```python
from build123d import *

# Parameters (mm, degrees)
F1_DEPTH = 2
F2_R     = 1
F3_R     = 4
F4_W     = 13.5
F4_H     = 1.8558323957
F5_DEPTH = 5
F6_R     = 1
F7_D     = 1


with BuildPart() as f1:
    # F0 (on Front) → F1 (new body)
    with BuildSketch(Plane.XZ):
        Polygon((5.5, 12.1071428571), (5.5, 7), (14, 7), (14, 20), align=None)
        Polygon((5.5, 12.1071428571), (0, 7), (5.5, 7), align=None)
        Polygon((5.5, 7), (0, 7), (0, -7.2836415662), (5.5, -7.188023068), align=None)
    extrude(amount=F1_DEPTH)

    # F2
    f2_edges = [f1.edges().sort_by_distance(p)[0] for p in [
        (0, -1, 7),
        (14, -1, 20),
        (14, -1, 7),
        (0, -1, -7.283642),
        (5.5, -1, -7.188023),
    ]]
    fillet(f2_edges, radius=F2_R)

    # F3
    f3_edges = [f1.edges().sort_by_distance(p)[0] for p in [
        (5.5, -1, 7),
    ]]
    fillet(f3_edges, radius=F3_R)

    # F4 (on Front) → F5 (join)
    with BuildSketch(Plane.XZ):
        with Locations((2.75, 0.9279161978)):
            Rectangle(F4_W, F4_H)
    extrude(amount=F5_DEPTH)

    # F6
    f6_edges = [f1.edges().sort_by_distance(p)[0] for p in [
        (9.5, -5, 0.927916),
        (-4, -5, 0.927916),
        (-4, 0, 0.927916),
        (9.5, 0, 0.927916),
    ]]
    fillet(f6_edges, radius=F6_R)

    # F7 (through all)
    with Locations(Plane(origin=(0, 0, 0), x_dir=(1, 0, 0), z_dir=(0, 1, 0))):
        with Locations((12.4978395179, -16.6222192347), (12.4978395179, -14.1531368718), (12.4978395179, -12.0000707684), (12.4978395179, -9.5441835001)):
            Hole(F7_D / 2)


solid = f1.part
```
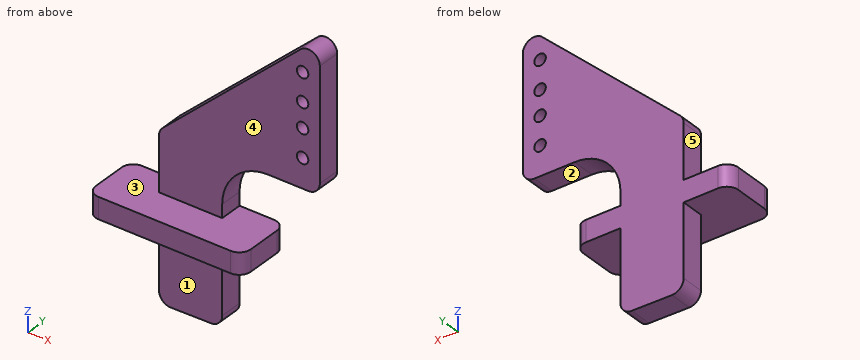
Geometry: final body of the model. Coordinates: model frame, mm. Face numbers are marked on the shaded views. A direction names the side the tool comes from. Give positions to 0.01 mm unless a question says otherwise; leave off trailing zeros. Write each loop counter-clockwise with the first axis right and the second up, starting at its lowest first coordinate (ties: lowest second). Pieces come first, ordered by that corner, then holes.
1. Section query D-D, the plane y = -2.7. Return loops of the section in (x, z).
2. Line query: probe 1 along Y at (x, z) = (2.5, -0.25); probe 2 along Z at (x, y) = (8.5, -4.35); probe 3 along X at (y, z) = (-1.3, 13.75). Output: solid intervals per line, ascending.
3. Section query B-B, the plane x = 7.25. Return loops of the section in (y, z).
4. Section query C-C, the plane y = -1.3. Return loops of the section in (x, z), then the cut area to 3 significant figures.
5. Reachability of the marked faces 1, 2, 3, 4 and 5 from +Z, -Z, +X, -X, +Y, -Y: full face, straight path, thin tool, end or side. Return the list, or none.
6. Pin query (flat end, axial travel): P1, Ø2, axis at y = -1, z = -3.5, coming from the -X side; P2, Ø1, axis at y = -3, z = 1, coming from the +X side; P3, Ø1.5, axis at x = 2.5, y = -2.5, coming from the -Z side. Return the tip coordinate at first contact, or that it passes through.
7. Section query A-A, the plane z = 0.75. Return loops of the section in (x, y).
Computed:
1. outline: (-4, 0) - (9.5, 0) - (9.5, 1.86) - (-4, 1.86) - close
2. probe 1: y = -2 to 0
2. probe 2: z = 0 to 1.86
2. probe 3: x = 7.27 to 12.2, 12.79 to 14
3. outline: (-5, 0) - (0, 0) - (0, 1.86) - (-5, 1.86) - close; (-2, 6.31) - (0, 6.31) - (0, 13.73) - (-2, 13.73) - close
4. outline: (-4, 0) - (0, 0) - (0, -6.27) arc R1 ccw to (1.02, -7.27) - (4.52, -7.21) arc R1 ccw to (5.5, -6.21) - (5.5, 0) - (9.5, 0) - (9.5, 1.86) - (5.5, 1.86) - (5.5, 3) arc R4 cw to (9.5, 7) - (13, 7) arc R1 ccw to (14, 8) - (14, 17.71) arc R1 ccw to (12.32, 18.44) - (0.32, 7.3) arc R1 ccw to (0, 6.56) - (0, 1.86) - (-4, 1.86) - close; hole circle Ø1 at (12.5, 9.54); hole circle Ø1 at (12.5, 12); hole circle Ø1 at (12.5, 14.15); hole circle Ø1 at (12.5, 16.62)
4. area: 183 mm2
5. face 1: -Z, +X, -X, -Y
5. face 2: -Z, +X, +Y, -Y
5. face 3: -Y
5. face 4: +Z, +X, -X, -Y
5. face 5: +Z, -X, +Y, -Y
6. P1: stops at x = 0
6. P2: stops at x = 9.5
6. P3: stops at z = -7.25
7. outline: (-4, -4) arc R1 ccw to (-3, -5) - (8.5, -5) arc R1 ccw to (9.5, -4) - (9.5, -1) arc R1 ccw to (8.5, 0) - (-3, 0) arc R1 ccw to (-4, -1) - close
